Verification items for the finished model (mm, model axes). Give positions to 0.01 mm unless a question says otherwise; leave off trailing zeros. Write each loop counter-clockwise with the first axis right and the second up, starting at its lowest first coordinate (ties: lowest second). Pieces come first, ordered by that corner, then holes. Notation, with made-up numbers: (40, 27) -> (98, 27) arc R16 ccw to (98, 31) -> close; hole circle Ø3 at (-17, -37.75). An arc over 180 degrees is marked (long way). Write item = value, one per line.
from build123d import *

# Parameters (mm, degrees)
SKETCH_1_W          = 15
SKETCH_1_H          = 15
SKETCH_1_W_2        = 13
SKETCH_1_H_2        = 13
EXTRUDE_1_DEPTH     = 394
SKETCH_2_R          = 1.45
SKETCH_2_R_2        = 1.65
CUT_EXTRUDE_1_DEPTH = 395.356754729
SKETCH_3_R          = 1.45
CUT_EXTRUDE_2_DEPTH = 395.356754729


with BuildPart() as part:
    # 草图1 → 凸台-拉伸1 (new body)
    with BuildSketch(Plane(origin=(0, 0, 0), x_dir=(0, 0, -1), z_dir=(1, 0, 0))):
        Rectangle(SKETCH_1_W, SKETCH_1_H)
        Rectangle(SKETCH_1_W_2, SKETCH_1_H_2, mode=Mode.SUBTRACT)
    extrude(amount=EXTRUDE_1_DEPTH)

    # 草图2 → 切除-拉伸1 (cut, through all)
    with BuildSketch(Plane(origin=(0, 7.5, 0), x_dir=(1, 0, 0), z_dir=(0, 1, 0))):
        with Locations(Location((380, 0, 0), (0, 0, 270))):
            Circle(SKETCH_2_R)
        with Locations(Location((370, 0, 0), (0, 0, 270))):
            Circle(SKETCH_2_R)
        with Locations(Location((196, 0, 0), (0, 0, 270))):
            Circle(SKETCH_2_R)
        with Locations(Location((206, 0, 0), (0, 0, 270))):
            Circle(SKETCH_2_R)
        with Locations(Location((8, 0, 0), (0, 0, 270))):
            Circle(SKETCH_2_R_2)
    extrude(amount=-CUT_EXTRUDE_1_DEPTH, mode=Mode.SUBTRACT)

    # 草图3 → 切除-拉伸2 (cut, through all)
    with BuildSketch(Plane.XY.offset(7.5)):
        with Locations((375, 0)):
            Circle(SKETCH_3_R)
        with Locations((385, 0)):
            Circle(SKETCH_3_R)
        with Locations((264, 0)):
            Circle(SKETCH_3_R)
        with Locations((254, 0)):
            Circle(SKETCH_3_R)
        with Locations((15, 0)):
            Circle(SKETCH_3_R)
    extrude(amount=-CUT_EXTRUDE_2_DEPTH, mode=Mode.SUBTRACT)


solid = part.part
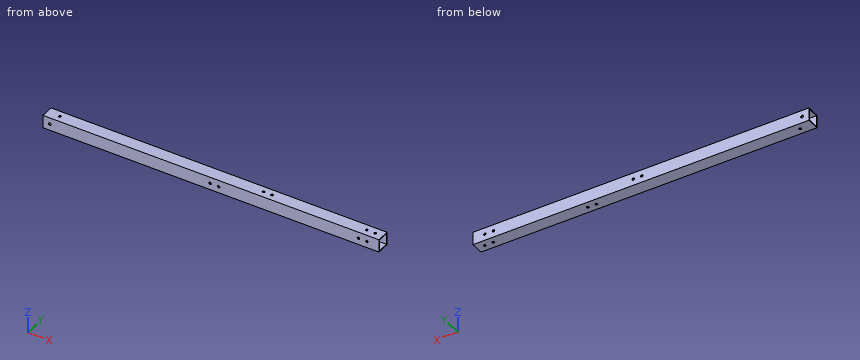
Item 1: Go/stop test with a flat-tipped pin: P1, Ø2.5, axis at x = 254, y = 0, coming from the +Z side (1 decimal). Record where the tip stops, or that it passes through.
Response values:
P1 = through
Item 2: Material ranges on line 1 (X direction, y = -7.1, z = 0); line 2 (Z direction, x = 221.5, y = -6.25), recorded low to high.
Response values:
line_1 = 0 to 6.35, 9.65 to 194.55, 197.45 to 204.55, 207.45 to 368.55, 371.45 to 378.55, 381.45 to 394
line_2 = -7.5 to -6.5, 6.5 to 7.5
Item 3: Sectioned sample at A-A on z = 4. Record the cut outline in (x, y).
Response values:
outline = (0, -7.5) -> (394, -7.5) -> (394, -6.5) -> (0, -6.5) -> close; (0, 6.5) -> (394, 6.5) -> (394, 7.5) -> (0, 7.5) -> close
Item 4: Sectioned sample at B-B on x = 275. Record the cut outline in (y, z).
Response values:
outline = (-7.5, -7.5) -> (7.5, -7.5) -> (7.5, 7.5) -> (-7.5, 7.5) -> close; hole (-6.5, -6.5) -> (6.5, -6.5) -> (6.5, 6.5) -> (-6.5, 6.5) -> close
